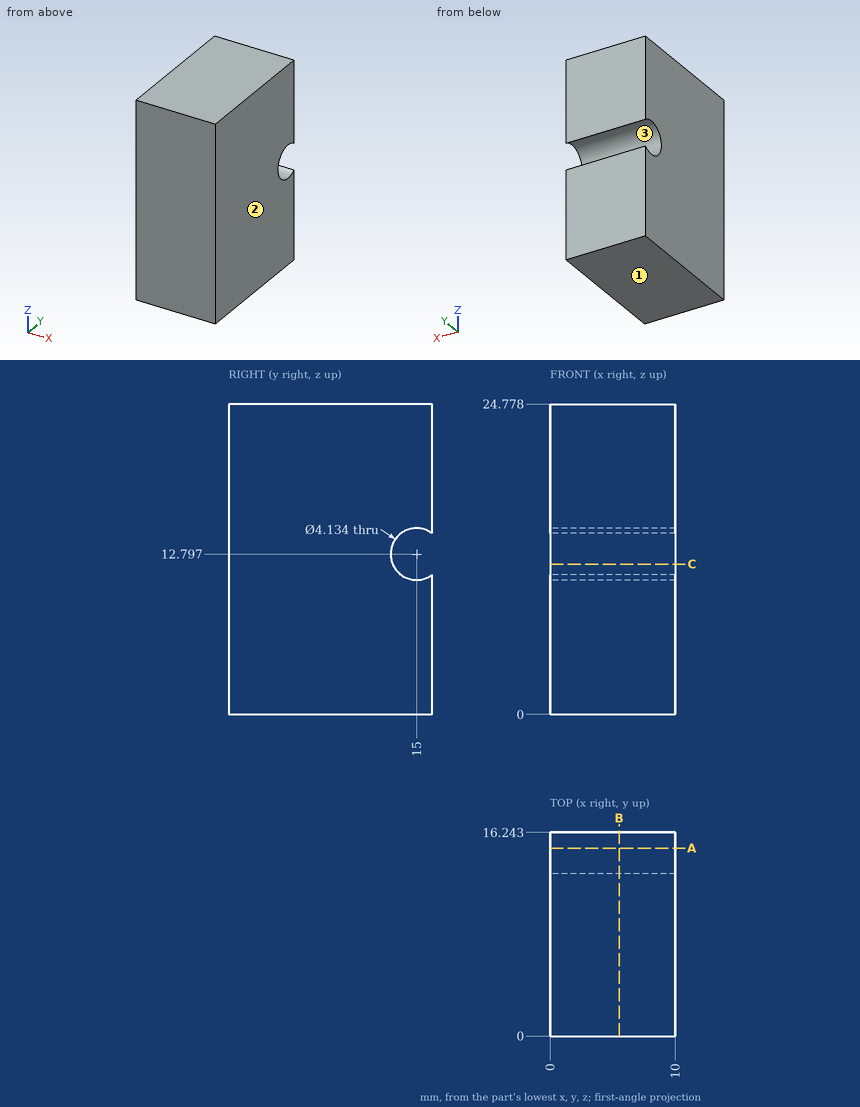
Part print with two shaded views. Sizes in mm from the minimum x, y, z corner. Coordinates: 2 decimals unless noted, no trailing zeros. Write each loop counter-clockwise with the first axis right and the second up, starting at its lowest first coordinate (ties: lowest second). Pieces come first, ordered by that corner, then holes. Notation, with made-up numbers: (41, -31.5) - (80, -31.5) arc R14 cw to (80, -12.5) - close; hole circle Ø6 at (17.5, 20). An arc over 180 degrees is marked (long way). Put each result on its own line as item: value.
1. Band-saw the part on B-B (x = 5.5). Write the cut outline in (y, z) (1 decimal).
Final values:
outline: (0, 0) - (16.2, 0) - (16.2, 11.1) arc R2.1 cw (long way) to (16.2, 14.4) - (16.2, 24.8) - (0, 24.8) - close
2. Two-plate mould, pull along Z, no slides. Class the marked faces 1, 2 and 3: +Z half, -Z half, draft (parallel to the pull), parting line (faces both ways), or undercut.
Final values:
face 1: -Z half
face 2: draft
face 3: undercut
3. Band-saw the part on A-A (y = 15). Write the cut outline in (x, z), then the cut area to 3 significant figures.
Final values:
outline: (0, 0) - (10, 0) - (10, 10.73) - (0, 10.73) - close; (0, 14.86) - (10, 14.86) - (10, 24.78) - (0, 24.78) - close
area: 206 mm²
4. Band-saw the part on C-C (z = 12). Write the cut outline in (x, y), then the cut area to 3 significant figures.
Final values:
outline: (0, 0) - (10, 0) - (10, 13.09) - (0, 13.09) - close
area: 131 mm²
5. Probe line 1 along Z through (x, y) = (4.5, 15); line 2 along Y through (x, z) = (1.25, 11); line 3 along Y through (x, z) = (2.5, 12.5). List the from-to ranges inside material, lowest first. Write a range as [from, to].
Final values:
line 1: z = [0, 10.73], [14.86, 24.78]
line 2: y = [0, 13.98], [16.02, 16.24]
line 3: y = [0, 12.95]
